Verification items for this drawing (mm, ordinates from the low corner). A direction names the side the tool comes from. Coordinates: 2 decimals unless noted, no trailing zeros. Write each loop counter-clockwise with the first axis right and the second up, starting at its lowest first coordinate (ties: lowest second). Pieces come first, ordered by that corner, then holes. Notation, with made-up numbers: (64, 50) -> (98, 50) arc R16 ccw to (98, 58) -> close; hole circle Ø1 at (-32.75, 30.25). An arc over 180 degrees is marked (long way). One line per question, with ' | ' between items.
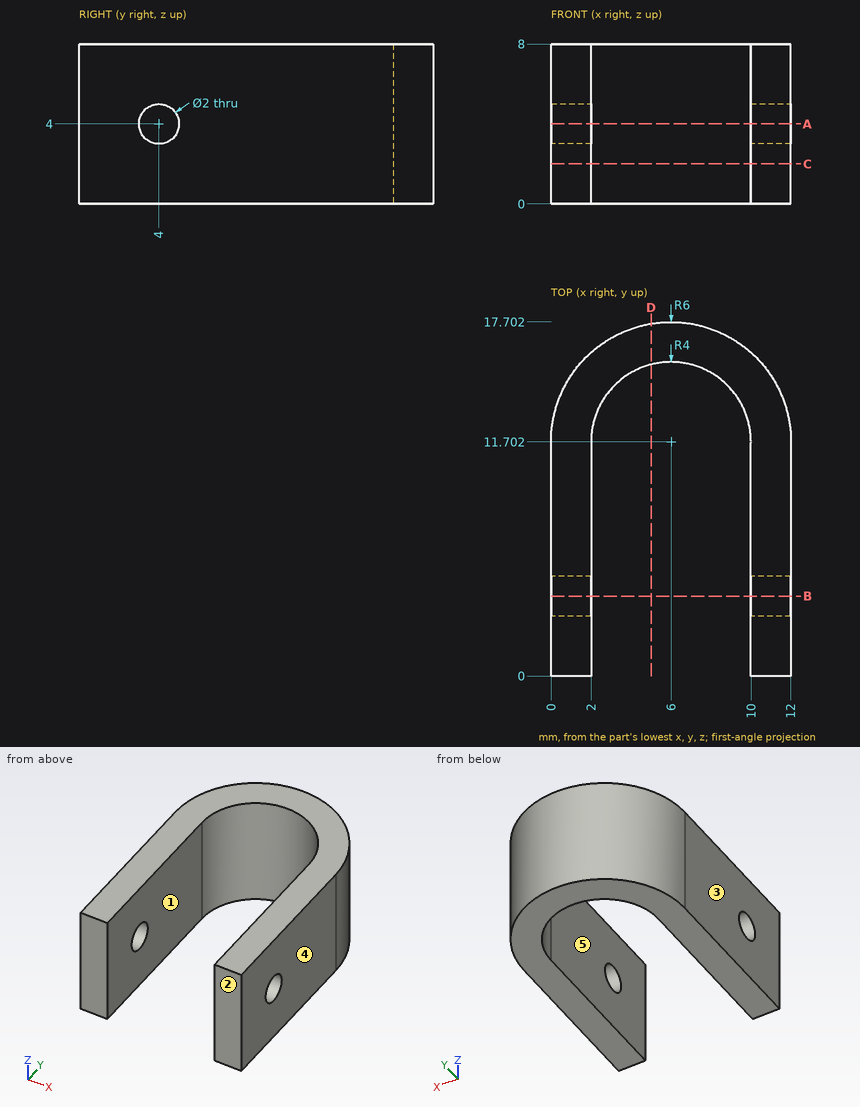
(1) Cross-section at B-B (y = 4). Record the cut outline in (x, z), plus the area to 3 significant figures.
Answers below:
outline: (0, 0) -> (2, 0) -> (2, 3) -> (0, 3) -> close; (0, 5) -> (2, 5) -> (2, 8) -> (0, 8) -> close; (10, 0) -> (12, 0) -> (12, 3) -> (10, 3) -> close; (10, 5) -> (12, 5) -> (12, 8) -> (10, 8) -> close | area: 24.0 mm²
(2) Tool access check on the marked faces 4 and 5. Record the directions out of +Z, -Z, +X, -X, +Y, -Y that give a thin tool (end or side, any length) a straight path to the whole face; none if there is none.
Answers below:
face 4: +Z, -Z, +X, +Y, -Y | face 5: +Z, -Z, -Y
(3) Draft check along X on the marked faces 1, 2 and 3. Enter one of: pulls with the +X half, pulls with the -X half, needs draft (parallel to the pull), parting line crosses it, or undercut.
Answers below:
face 1: undercut | face 2: needs draft | face 3: pulls with the -X half
(4) Cross-section at A-A (z = 4). Record the cut outline in (x, y).
Answers below:
outline: (0, 0) -> (2, 0) -> (2, 3) -> (0, 3) -> close; (0, 5) -> (2, 5) -> (2, 11.7) arc R4 cw to (10, 11.7) -> (10, 5) -> (12, 5) -> (12, 11.7) arc R6 ccw to (0, 11.7) -> close; (10, 0) -> (12, 0) -> (12, 3) -> (10, 3) -> close
(5) Depth check by flat-ended pin: P1, Ø1.6, axis at y = 4, z = 4, coming from the -X side; P2, Ø1, axis at y = 12.5, z = 1, coming from the +X side. Enter the tip coordinate at first touch or a pass-through.
Answers below:
P1: passes through | P2: stops at x = 11.99
(6) Material ranges on line 1 (X direction, y = 4.25, z = 3); line 2 (Y direction, x = 10.95, z = 4) (1 decimal); line 3 (Y direction, x = 11.05, z = 4) (1 decimal), recorded low to high.
Answers below:
line 1: x = 0 to 2, 10 to 12 | line 2: y = 0 to 3, 5 to 15.1 | line 3: y = 0 to 3, 5 to 14.9
(7) Cross-section at C-C (z = 2). Record the cut outline in (x, y).
Answers below:
outline: (0, 0) -> (2, 0) -> (2, 11.7) arc R4 cw to (10, 11.7) -> (10, 0) -> (12, 0) -> (12, 11.7) arc R6 ccw to (0, 11.7) -> close
(8) Cross-section at D-D (x = 5). Record the cut outline in (y, z) (1 decimal).
Answers below:
outline: (15.6, 0) -> (17.6, 0) -> (17.6, 8) -> (15.6, 8) -> close
